Can you work these out from the model? Positions are in its coordinate system, mm. Face numbers are marked on the shaded views. A direction names the side the tool comes from. Coordinates: 2 decimals unless noted, no trailing zeros. Order: outer loops, then holes, each group sorted by start corner. A loop starts at its lowest first (then second) coordinate and runs counter-clockwise, first axis right, second up. Notation, with made-up numbers: (55.5, 85) -> (104.5, 85) arc R17 cw to (104.5, 99) -> close; hole circle Ø9 at (-15.5, 73). An arc over 180 degrees is marked (long way). Answer in a Markdown table with one row per item. Add a question column.
1. If I drill on line 1 along X through (y, z) = (30.1, -4.9); line 2 along Z through (x, y) = (24, 29.8); line 3 along X through (y, z) = (16, 0.25), over which ranges is the centre line in solid material (lowest first)? Write a range as [from, to].
2. Imagine slicing it at A-A on z = 4.9. Write out the boundary of the cut face in (x, y), plus the area to 3 significant figures.
3. Imagine slicing it at B-B on x = -24. Write out the boundary of the cut face in (y, z).
4. On a 3-axis mill with a long thin cutter (end or side, diameter ignored), from which of +Z, -Z, +X, -X, +Y, -Y can I reach the whole of each face in a straight line? I mean the marked faces 1, 2 and 3. Say none if no direction works.
5. Will these pins go through, and if not, where does the flat tip stop? pin 1 (2 mm diameter, centred on x = 23.5, z = 4, fed in from +Y); pin 2 (5 mm diameter, centred on x = -24, z = -4.9, fed in from -Y); pin 3 (2.5 mm diameter, centred on y = 34.5, z = 2.5, fed in from +X); pin 4 (6.5 mm diameter, centred on y = 35.5, z = -0.5, fed in from -X).
6. Imagine slicing it at C-C on z = 0. Write out the boundary of the cut face in (x, y), plus the area to 3 significant figures.
7. Imagine slicing it at D-D on x = -12. Write out the boundary of the cut face in (y, z), plus the area to 3 significant figures.
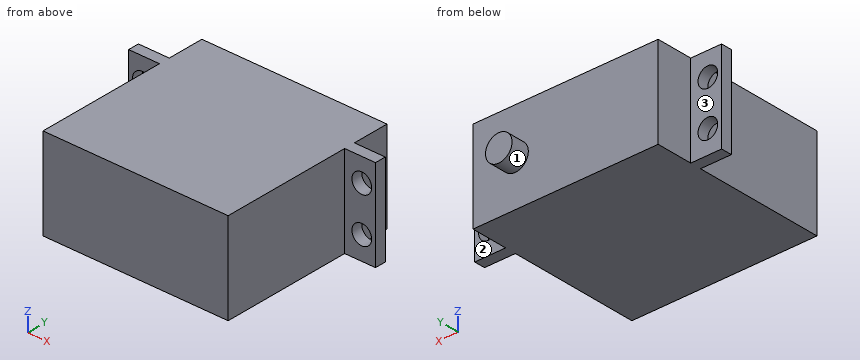
from build123d import *

# Parameters (mm, degrees)
SKETCH_1_W          = 40.5
SKETCH_1_H          = 20
EXTRUDE_1_DEPTH     = 28.6
SKETCH_2_W          = 54
SKETCH_2_H          = 20
EXTRUDE_2_DEPTH     = 2.4
SKETCH_3_W          = 40.5
SKETCH_3_H          = 20
EXTRUDE_3_DEPTH     = 8
SKETCH_4_R          = 2.9
EXTRUDE_4_DEPTH     = 4
SKETCH_5_R          = 2.15
CUT_EXTRUDE_1_DEPTH = 32


with BuildPart() as part:
    # 草图1 → 凸台-拉伸1 (new body)
    with BuildSketch(Plane(origin=(0, 0, 0), x_dir=(1, 0, 0), z_dir=(0, 1, 0))):
        Rectangle(SKETCH_1_W, SKETCH_1_H)
    extrude(amount=EXTRUDE_1_DEPTH)

    # 草图2 → 凸台-拉伸2 (add)
    with BuildSketch(Plane(origin=(0, 28.6, 0), x_dir=(1, 0, 0), z_dir=(0, 1, 0))):
        Rectangle(SKETCH_2_W, SKETCH_2_H)
    extrude(amount=EXTRUDE_2_DEPTH)

    # 草图3 → 凸台-拉伸3 (add)
    with BuildSketch(Plane(origin=(0, 31, 0), x_dir=(1, 0, 0), z_dir=(0, 1, 0))):
        Rectangle(SKETCH_3_W, SKETCH_3_H)
    extrude(amount=EXTRUDE_3_DEPTH)

    # 草图4 → 凸台-拉伸4 (add)
    with BuildSketch(Plane(origin=(0, 39, 0), x_dir=(1, 0, 0), z_dir=(0, 1, 0))):
        with Locations((11.05, 0)):
            Circle(SKETCH_4_R)
    extrude(amount=EXTRUDE_4_DEPTH)

    # 草图5 → 切除-拉伸1 (cut, through all)
    with BuildSketch(Plane(origin=(0, 31, 0), x_dir=(1, 0, 0), z_dir=(0, 1, 0))):
        with Locations((24, 4.9)):
            Circle(SKETCH_5_R)
        with Locations((24, -4.9)):
            Circle(SKETCH_5_R)
        with Locations((-24, -4.9)):
            Circle(SKETCH_5_R)
        with Locations((-24, 4.9)):
            Circle(SKETCH_5_R)
    extrude(amount=-CUT_EXTRUDE_1_DEPTH, mode=Mode.SUBTRACT)


solid = part.part
Answers follow:
| question | item | result |
|---|---|---|
| 1 | line 1 | x = [-27, -26.15], [-21.85, 21.85], [26.15, 27] |
| 1 | line 2 | z = [-10, -7.05], [-2.75, 2.75], [7.05, 10] |
| 1 | line 3 | x = [-20.25, 20.25] |
| 2 | outline | (-27, 28.6) -> (-26.15, 28.6) -> (-26.15, 31) -> (-27, 31) -> close; (-21.85, 28.6) -> (-20.25, 28.6) -> (-20.25, 0) -> (20.25, 0) -> (20.25, 28.6) -> (21.85, 28.6) -> (21.85, 31) -> (20.25, 31) -> (20.25, 39) -> (-20.25, 39) -> (-20.25, 31) -> (-21.85, 31) -> close; (26.15, 28.6) -> (27, 28.6) -> (27, 31) -> (26.15, 31) -> close |
| 2 | area | 1,590 mm² |
| 3 | outline | (28.6, -10) -> (31, -10) -> (31, -7.05) -> (28.6, -7.05) -> close; (28.6, -2.75) -> (31, -2.75) -> (31, 2.75) -> (28.6, 2.75) -> close; (28.6, 7.05) -> (31, 7.05) -> (31, 10) -> (28.6, 10) -> close |
| 4 | face 1 | +Y |
| 4 | face 2 | +Z, -Z, +X, +Y |
| 4 | face 3 | +Z, -Z, -X, +Y |
| 5 | pin 1 | passes through |
| 5 | pin 2 | stops at y = 28.6 |
| 5 | pin 3 | stops at x = 20.25 |
| 5 | pin 4 | stops at x = -20.25 |
| 6 | outline | (-27, 28.6) -> (-20.25, 28.6) -> (-20.25, 0) -> (20.25, 0) -> (20.25, 28.6) -> (27, 28.6) -> (27, 31) -> (20.25, 31) -> (20.25, 39) -> (13.95, 39) -> (13.95, 43) -> (8.15, 43) -> (8.15, 39) -> (-20.25, 39) -> (-20.25, 31) -> (-27, 31) -> close |
| 6 | area | 1,640 mm² |
| 7 | outline | (0, -10) -> (39, -10) -> (39, 10) -> (0, 10) -> close |
| 7 | area | 780 mm² |
